Part model, mm, in its own coordinate system. A direction names the side the tool comes from. Coordinates: 2 decimals unless noted, no trailing zeros. Loops run counter-clockwise (first coordinate to the right, second up) from the corner with the lowest first, then second, coordinate; pieces in that order, holes last. Notation, with made-up numbers: M 9.5,-29.75 L 44.5,-29.75 A12 cw 44.5,-19.75 Z; hole C -36,-5 d7. An arc over 180 degrees is marked long. Use a Markdown table: item, result. Add a question column.
1) Wall check: probe 1 along Y at (x, z) = (13, 2.75); probe 2 along Y at (x, z) = (30, 0.45); probe 3 along Y at (x, z) = (-10, 0.4). Give the ranges that are in metal, low to high. Write a range as from..to.
2) Pin check, flat tips, straight feed: pin 1 Ø1.8 at (y, z) = (2, 0.5) entering from -X; pin 2 Ø2 at (x, z) = (-7.5, 1.5) entering from +Y; pin 3 Ø1.6 at (x, y) = (0, -9.87) entering from -Z; pin 4 Ø3 at (y, z) = (1, -0.5) entering from +X. Stop position of each tip, or through.
3) Band-saw the part on A-A (x = 12.5). List the corners of the cut face in (y, z), plus the area to 3 significant figures.
4) Band-saw the part on B-B (y = -27). List the corners of the cut face in (x, z), plus the area to 3 significant figures.
5) Band-saw the part on C-C (z = -2). State how many separate pieces and enclosed holes the cut face has, plus the area to 3 significant figures.
6) Tool access for faces 4 (the flat face through (26.578, -24.354, 0.042)), 5 (the flat face through (8.55, 1, 0)), 6 (the flat face through (14, 4.936, 0)): list every direction of +Z, -Z, +X, -X, +Y, -Y with a clear straight run to the whole face (end or side of a thin tool).
7) Pull direction X, two halves, no side cores. Call faces 1 (the flat face through (10, -11, -3)), 2 (the cylindrical face through (-11.852, -31.941, -0.042)), 3 (the flat face through (-17.972, 2.964, 0.042)): released by +X, released by -X, zero draft, split by the parting line, or undercut.
8) Band-saw the part on D-D (y = -42.5). List the corners of the cut face in (x, z), plus the area to 3 significant figures.
from build123d import *

# Parameters (mm, degrees)
SKETCH_1_R          = 2.1
EXTRUDE_1_DEPTH     = 3
CHAMFER_1_SIZE      = 4
SKETCH_2_R          = 1
CUT_EXTRUDE_1_DEPTH = 67.274052238
CUT_EXTRUDE_2_DEPTH = 67.274052238
FILLET_1_R          = 2
CHAMFER_2_SIZE      = 2


with BuildPart() as part:
    # 草图1 → 凸台-拉伸1 (new, symmetric)
    with BuildSketch(Plane.XY):
        Polygon((-20, 4.936344802), (-20, -52.5), (40, -52.5), (40, -32.5), (20, 4.936344802), (8.55, 4.936344802), (8.55, -4.936344802), (0, -9.872689603), (-8.55, -4.936344802), (-8.55, 4.936344802), align=None)
        with Locations((-10, -42.5)):
            Circle(SKETCH_1_R, mode=Mode.SUBTRACT)
        with Locations((30, -42.5)):
            Circle(SKETCH_1_R, mode=Mode.SUBTRACT)
    extrude(amount=EXTRUDE_1_DEPTH, both=True)

    # 倒角1
    chamfer_1_edges = [part.edges().sort_by_distance(p)[0] for p in [
        (40, -52.5, 0),
        (-20, -52.5, 0),
        (-20, 4.936344802, 0),
    ]]
    chamfer(chamfer_1_edges, length=CHAMFER_1_SIZE)

    # 草图2 → 切除-拉伸1 (cut, through all)
    with BuildSketch(Plane.XY.offset(3)):
        with Locations((-8.05, -4.070319398)):
            Circle(SKETCH_2_R)
        with Locations((8.05, -4.070319398)):
            Circle(SKETCH_2_R)
        with Locations((0, -9.872689603)):
            Circle(SKETCH_2_R)
    extrude(amount=-CUT_EXTRUDE_1_DEPTH, mode=Mode.SUBTRACT)

    # 草图3 → 切除-拉伸2 (cut, through all)
    with BuildSketch(Plane.XY.offset(3)):
        Polygon((-12, -15.872689603), (-12, -32.014718626), (0.485281374, -44.5), (19.514718626, -44.5), (31.133551708, -32.881166917), (22.046939538, -15.872689603), align=None)
    extrude(amount=-CUT_EXTRUDE_2_DEPTH, mode=Mode.SUBTRACT)

    # 圆角1
    fillet_1_edges = [part.edges().sort_by_distance(p)[0] for p in [
        (-12, -15.872689603, 0),
        (22.046939538, -15.872689603, 0),
        (31.133551708, -32.881166917, 0),
        (19.514718626, -44.5, 0),
        (0.485281374, -44.5, 0),
        (-12, -32.014718626, 0),
    ]]
    fillet(fillet_1_edges, radius=FILLET_1_R)

    # 倒角2
    chamfer_2_edges = [part.edges().sort_by_distance(p)[0] for p in [
        (-12.1, -42.5, -3),
        (27.9, -42.5, -3),
    ]]
    chamfer(chamfer_2_edges, length=CHAMFER_2_SIZE)


solid = part.part
Entries:
| question | item | result |
|---|---|---|
| 1 | probe 1 | -52.5..-44.5, -15.87..4.94 |
| 1 | probe 2 | -52.5..-44.6, -40.4..-34.01, -30.76..-13.78 |
| 1 | probe 3 | -52.5..-44.6, -40.4..-34.01, -15.87..4.94 |
| 2 | pin 1 | x = -19.84 |
| 2 | pin 2 | y = -4.97 |
| 2 | pin 3 | through |
| 2 | pin 4 | x = 22.9 |
| 3 | outline | M -52.5,-3 L -44.5,-3 L -44.5,3 L -52.5,3 Z; M -15.87,-3 L 4.94,-3 L 4.94,3 L -15.87,3 Z |
| 3 | area | 173 mm2 |
| 4 | outline | M -20,-3 L -12,-3 L -12,3 L -20,3 Z; M 27.99,-3 L 37.06,-3 L 37.06,3 L 27.99,3 Z |
| 4 | area | 102 mm2 |
| 5 | separate pieces | 1 |
| 5 | enclosed holes | 3 |
| 5 | area | 1,760 mm2 |
| 6 | face 4 | +Z, -Z |
| 6 | face 5 | +Z, -Z, +Y |
| 6 | face 6 | +Z, -Z, +X, -X, +Y |
| 7 | face 1 | zero draft |
| 7 | face 2 | undercut |
| 7 | face 3 | released by -X |
| 8 | outline | M -20,-3 L -14.1,-3 L -12.1,-1 L -12.1,3 L -20,3 Z; M -7.9,-1 L -5.9,-3 L -1.51,-3 L -1.51,3 L -7.9,3 Z; M 21.51,-3 L 25.9,-3 L 27.9,-1 L 27.9,3 L 21.51,3 Z; M 32.1,-1 L 34.1,-3 L 40,-3 L 40,3 L 32.1,3 Z |
| 8 | area | 163 mm2 |
